from build123d import *

# Parameters (mm, degrees)
SKETCH1_R           = 40.64
BOSS_EXTRUDE1_DEPTH = 3.683
SKETCH10_R          = 1.5875
CUT_EXTRUDE3_DEPTH  = 4.683
SKETCH12_R          = 1.5875
CUT_EXTRUDE4_DEPTH  = 4.683
SKETCH13_R          = 3.81
SKETCH13_R_2        = 1.5875
BOSS_EXTRUDE2_DEPTH = 3.175
FILLET1_R           = 0.508


with BuildPart() as part:
    # Sketch1 → Boss-Extrude1 (new body)
    with BuildSketch(Plane(origin=(0, 0, 0), x_dir=(0, 0, -1), z_dir=(1, 0, 0))):
        Circle(SKETCH1_R)
    extrude(amount=BOSS_EXTRUDE1_DEPTH)

    # Sketch10 → Cut-Revolve1 (revolve, cut)
    with BuildSketch(Plane.XY):
        with Locations((1.8415, 40.64)):
            Circle(SKETCH10_R)
    revolve(axis=Axis((-1.01619145, 0, 0), (1, 0, 0)), mode=Mode.SUBTRACT)

    # Sketch11 → Cut-Extrude3 (cut, through all)
    with BuildSketch(Plane(origin=(3.683, 0, 0), x_dir=(0, 0, -1), z_dir=(1, 0, 0))):
        with BuildLine():
            Line((-1.27, 36.172712436), (-1.27, 6.221703947))
            ThreePointArc((-1.27, 6.221703947), (-2.430039796, 5.866635031), (-3.501383439, 5.297434663))
            Line((-3.501383439, 5.297434663), (-24.679944646, 26.47599587))
            ThreePointArc((-24.679944646, 26.47599587), (-13.851226834, 33.439819679), (-1.27, 36.172712436))
        make_face()
        with BuildLine():
            Line((1.27, 36.172712436), (1.27, 6.221703947))
            ThreePointArc((1.27, 6.221703947), (2.430039796, 5.866635031), (3.501383439, 5.297434663))
            Line((3.501383439, 5.297434663), (24.679944646, 26.47599587))
            ThreePointArc((24.679944646, 26.47599587), (13.851226834, 33.439819679), (1.27, 36.172712436))
        make_face()
        with BuildLine():
            Line((26.47599587, 24.679944646), (5.297434663, 3.501383439))
            ThreePointArc((5.297434663, 3.501383439), (5.866635031, 2.430039796), (6.221703947, 1.27))
            Line((6.221703947, 1.27), (36.172712436, 1.27))
            ThreePointArc((36.172712436, 1.27), (33.439819679, 13.851226834), (26.47599587, 24.679944646))
        make_face()
        with BuildLine():
            Line((36.172712436, -1.27), (6.221703947, -1.27))
            ThreePointArc((6.221703947, -1.27), (5.866635031, -2.430039796), (5.297434663, -3.501383439))
            Line((5.297434663, -3.501383439), (26.47599587, -24.679944646))
            ThreePointArc((26.47599587, -24.679944646), (33.439819679, -13.851226834), (36.172712436, -1.27))
        make_face()
        with BuildLine():
            Line((24.679944646, -26.47599587), (3.501383439, -5.297434663))
            ThreePointArc((3.501383439, -5.297434663), (2.430039796, -5.866635031), (1.27, -6.221703947))
            Line((1.27, -6.221703947), (1.27, -36.172712436))
            ThreePointArc((1.27, -36.172712436), (13.851226834, -33.439819679), (24.679944646, -26.47599587))
        make_face()
        with BuildLine():
            Line((-1.27, -36.172712436), (-1.27, -6.221703947))
            ThreePointArc((-1.27, -6.221703947), (-2.430039796, -5.866635031), (-3.501383439, -5.297434663))
            Line((-3.501383439, -5.297434663), (-24.679944646, -26.47599587))
            ThreePointArc((-24.679944646, -26.47599587), (-13.851226834, -33.439819679), (-1.27, -36.172712436))
        make_face()
        with BuildLine():
            Line((-26.47599587, -24.679944646), (-5.297434663, -3.501383439))
            ThreePointArc((-5.297434663, -3.501383439), (-5.866635031, -2.430039796), (-6.221703947, -1.27))
            Line((-6.221703947, -1.27), (-36.172712436, -1.27))
            ThreePointArc((-36.172712436, -1.27), (-33.439819679, -13.851226834), (-26.47599587, -24.679944646))
        make_face()
        with BuildLine():
            Line((-36.172712436, 1.27), (-6.221703947, 1.27))
            ThreePointArc((-6.221703947, 1.27), (-5.866635031, 2.430039796), (-5.297434663, 3.501383439))
            Line((-5.297434663, 3.501383439), (-26.47599587, 24.679944646))
            ThreePointArc((-26.47599587, 24.679944646), (-33.439819679, 13.851226834), (-36.172712436, 1.27))
        make_face()
    extrude(amount=-CUT_EXTRUDE3_DEPTH, mode=Mode.SUBTRACT)

    # Sketch12 → Cut-Extrude4 (cut, through all)
    with BuildSketch(Plane(origin=(3.683, 0, 0), x_dir=(0, 0, -1), z_dir=(1, 0, 0))):
        Circle(SKETCH12_R)
    extrude(amount=-CUT_EXTRUDE4_DEPTH, mode=Mode.SUBTRACT)

    # Sketch13 → Boss-Extrude2 (add)
    with BuildSketch(Plane(origin=(3.683, 0, 0), x_dir=(0, 0, -1), z_dir=(1, 0, 0))):
        Circle(SKETCH13_R)
        Circle(SKETCH13_R_2, mode=Mode.SUBTRACT)
    extrude(amount=BOSS_EXTRUDE2_DEPTH)

    # Fillet1
    fillet1_edges = [part.edges().sort_by_distance(p)[0] for p in [
        (3.683, 0, 3.81),
    ]]
    fillet(fillet1_edges, radius=FILLET1_R)


solid = part.part
Design review of the part built by this model. Coordinates are the model's own, in mm. A direction names the side the tool comes from. Give positions to 0.01 mm unless a question says otherwise; leave off trailing zeros. Answer as a JSON object with one key per item and string values.
Item 1: Wall thickness on line 1 along Y through (x, z) = (1.75, -19); line 2 along Z through (x, y) = (3.5, 13); line 3 along Y through (x, z) = (2.5, -7): over which ranges is each line inside the solid? List them lowest first.
Output values:
{"line 1": "y = -34.12 to -30.81, -20.8 to -17.2, -1.27 to 1.27, 17.2 to 20.8, 30.81 to 34.12", "line 2": "z = -38.5 to -33.78, -14.8 to -11.2, -1.27 to 1.27, 11.2 to 14.8, 33.78 to 38.5", "line 3": "y = -38.57 to -35.51, -8.8 to -5.2, -1.27 to 1.27, 5.2 to 8.8, 35.51 to 38.57"}
Item 2: Machinability: for faces 4 (the face through (1.87, -14.02, -33.37)), 5 (the face through (0, -8, 1)), which of the approach directions +Z, -Z, +X, -X, +Y, -Y give a long, thin tool a straight path to every point of the face, cutting with its end or side? Answer none if there is none.
Output values:
{"face 4": "+X, -X", "face 5": "+Z, -Z, -X, +Y, -Y"}
Item 3: We need section C-C (x = 1.5). Count the separate pieces of the cut face and the enclosed holes in it, and give its area (3 significant figures).
Output values:
{"separate pieces": "1", "enclosed holes": "9", "area": "1,410 mm2"}
Item 4: Mouldability with a two-part tool opening along Y and no side actions: class faces 1 (the face through (5.51, -3.72, 0.83)), 2 (the face through (2, -1.27, 21)), 3 (the face through (6.858, 0, -2)) as pulls with the +Y half, pulls with the -Y half, needs draft (parallel to the pull), parting line crosses it, or undercut.
Output values:
{"face 1": "parting line crosses it", "face 2": "undercut", "face 3": "needs draft"}
Item 5: For P1, Ø1.1, axis at x = 2.5, z = 18, coming from the -Y side; P2, Ø10, axis at y = 15.5, z = 6.5, coming from the +X side (1 decimal); P3, Ø1.8, axis at x = 1.5, z = -22, coming from the -Y side; P4, Ø1.1, axis at x = 2, y = 14, coming from the +Z side, all flat-tipped, find the tip position at first contact; note any pin that passes through.
Output values:
{"P1": "stops at y = -35.34", "P2": "passes through", "P3": "stops at y = -33.12", "P4": "stops at z = 36.71"}
